Part model, mm, in its own coordinate system. Face numbers are marked on the shaded views. Give positions to 0.01 mm unless a question says otherwise; leave off trailing zeros. Loops run counter-clockwise (first coordinate to the right, second up) from the corner with the lowest first, then second, coordinate; pieces in that order, holes last. Notation, with made-up numbers: M 89.25,75 L 127.25,75 A26 ccw 127.25,93 Z; hole C 51,1 d1. An arc over 180 degrees is marked long. Answer in a Markdown table with one row per item.
from build123d import *

# Parameters (mm, degrees)
F0_R      = 25
F1_DEPTH  = 200
F2_R      = 20
F3_DEPTH  = 65
F4_W      = 10
F4_H      = 3.1937984634
F5_DEPTH  = 61.7
F7_D      = 24.16
F7_DEPTH  = 75
F7_TIP    = 7.2583962779
F8_W      = 10
F8_H      = 5.6645046324
F9_DEPTH  = 70
F11_R     = 2
F12_DEPTH = 25
F13_R     = 3.75
F14_DEPTH = 6


with BuildPart() as f1:
    # F0 (on Front) → F1 (new body)
    with BuildSketch(Plane.XZ):
        Circle(F0_R)
    extrude(amount=F1_DEPTH)

    # F2 (on face) → F3 (join)
    with BuildSketch(Plane.XZ.offset(200)):
        Circle(F2_R)
    extrude(amount=F3_DEPTH)

    # F4 (on face) → F5 (cut)
    with BuildSketch(Plane.XZ.offset(265)):
        with Locations((0, 20.9618159628)):
            Rectangle(F4_W, F4_H)
    extrude(amount=-F5_DEPTH, mode=Mode.SUBTRACT)

    # F7
    with Locations(Plane(origin=(0, 0, 0), x_dir=(-1, 0, 0), z_dir=(0, 1, 0))):
        with Locations((0, 0)):
            Hole(F7_D / 2, depth=F7_DEPTH)
            with Locations((0, 0, -(F7_DEPTH + F7_TIP / 2))):  # 118° drill point
                Cone(0, F7_D / 2, F7_TIP, mode=Mode.SUBTRACT)

    # F8 (on face) → F9 (cut)
    with BuildSketch(Plane(origin=(0, 0, 0), x_dir=(-1, 0, 0), z_dir=(0, 1, 0))):
        with Locations((0, 11.6677476838)):
            Rectangle(F8_W, F8_H)
    extrude(amount=-F9_DEPTH, mode=Mode.SUBTRACT)

    # F11 (on offset) → F12 (cut)
    with BuildSketch(Plane.XY.offset(25)):
        with Locations((0, -35)):
            Circle(F11_R)
    extrude(amount=-F12_DEPTH, mode=Mode.SUBTRACT)

    # F13 (on offset) → F14 (cut)
    with BuildSketch(Plane.XY.offset(25)):
        with Locations((0, -34.9959954619)):
            Circle(F13_R)
    extrude(amount=-F14_DEPTH, mode=Mode.SUBTRACT)


solid = f1.part
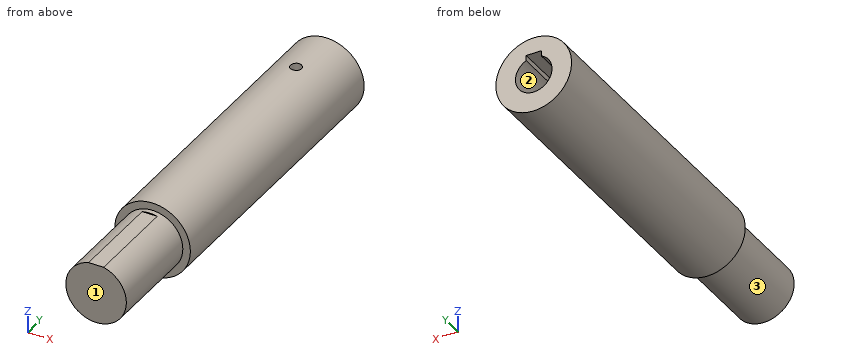
(1) Pin check, flat tips, straight feed: pin 1 Ø12 at (x, y) = (-15, -211.5) entering from -Z; pin 2 Ø12 at (x, y) = (0, -35) entering from -Z; pin 3 Ø12 at (x, y) = (14, -84.5) entering from +Z. Stop position of each tip, or through.
Recorded:
| item | result |
|---|---|
| pin 1 | stops at z = -17.86 |
| pin 2 | stops at z = -25 |
| pin 3 | stops at z = 23.69 |
(2) Saw through at B-B (y = -101). Write the cut outline in (x, z).
Recorded:
| item | result |
|---|---|
| outline | C 0,0 d50 |
(3) Drill centre lines: line 1 along Y through (x, z) = (0, 23.25); line 2 along Z through (x, y) = (0, -45.5); line 3 along Z through (x, y) = (0, -35). Where is each one in solid material? Low to high.
Recorded:
| item | result |
|---|---|
| line 1 | y = -200 to -38.75, -31.25 to 0 |
| line 2 | z = -25 to -12.08, 14.5 to 25 |
| line 3 | z = -25 to -12.08 |
(4) Saw through at C-C (y = -215.5). Write the cut outline in (x, z), plus the area to 3 significant figures.
Recorded:
| item | result |
|---|---|
| outline | M -5,19.36 A20 ccw long 5,19.36 Z |
| area | 1,250 mm^2 |
(5) Saw through at A-A (z = -17.5). Write the cut outline in (x, y), plus the area to 3 significant figures.
Recorded:
| item | result |
|---|---|
| outline | M -17.85,-200 L -9.68,-200 L -9.68,-265 L 9.68,-265 L 9.68,-200 L 17.85,-200 L 17.85,0 L -17.85,0 Z |
| area | 8,400 mm^2 |
(6) Pull direction X, two halves, no side cores. Call the marked faces 1, 2 and 3: +X half, -X half, draft (parallel to the pull), parting line (faces both ways), or undercut.
Recorded:
| item | result |
|---|---|
| face 1 | draft |
| face 2 | undercut |
| face 3 | parting line |
